Can you work these out from the model? Positions are in its coordinate system, mm. A direction names the side the tool comes from. Round coordinates to 2 decimals unless told otherwise and drop trailing zeros. Write each loop counter-clockwise with the first axis right and the second up, starting at its lowest first coordinate (ties: lowest second). Pieces come first, ordered by that corner, then holes. Notation, with made-up numbers: M 83.5,-25.75 L 109.5,-25.75 A21 cw 109.5,-2.75 Z; hole C 40,34.25 d5. An arc over 180 degrees is marked long. Answer in a Markdown table with one row per item. Add a question column.
(1) Suppose I cut it at B-B, the plane z = 5.3. Write out the boundary of the cut face in (x, y), then the cut area to 3 significant figures.
(2) If I drill on probe 1 along Y at (x, z) = (0, 3.75); probe 2 along Y at (x, z) = (0, 5.75); probe 3 along Z at (x, y) = (-0.2, -17), over which ranges is the centre line in solid material (lowest first)?
(3) If we mould it in two halves opening along X, with no side actions, what happens to faces 1 (the face through (-0.014, -16.405, 4.844)), 2 (the face through (1, 16, 5)), 3 (the face through (5.65, -1.03, 3.79))? For each: released by +X, released by -X, zero draft, split by the parting line, or undercut.
(4) I'm going to push flat-ended pins straight in: pin 1 (2.5 mm diameter, centred on x = 0, y = -6, fed in from +Z); pin 2 (3 mm diameter, centred on x = 0, y = 7, fed in from +Z); pin 3 (2 mm diameter, centred on y = -7.5, z = 5.5, fed in from +X); pin 4 (1.7 mm diameter, centred on y = 17, z = 5.3, fed in from +X). Where does each tip first touch, or does it pass through?
(5) For faces 4 (the face through (15, 0, 7)), 5 (the face through (-1, -16, 5)), 6 (the face through (0.585, -4.364, 6.279)), which set-ups out of +Z, -Z, +X, -X, +Y, -Y let a thin tool reach every point of the face, with its end or its side?
(6) Suppose I cut it at A-A, the plane x = 0. Write out the boundary of the cut face in (y, z).
from build123d import *

# Parameters (mm, degrees)
SKETCH050_R             = 15
SKETCH050_R_2           = 2.75
SKETCH050_R_3           = 1.7
PAD021_DEPTH            = 5
SKETCH051_R             = 2.7
POCKET026_DEPTH         = 88.441037
POLARPATTERN004_COUNT   = 4
PAD022_DEPTH            = 5
SKETCH054_R             = 0.75
POCKET027_DEPTH         = 5
POLARPATTERN005_COUNT   = 2
BODY011_PLACEMENT_ANGLE = 270


with BuildPart() as part:
    # Sketch050 → Pad021 (new body)
    with BuildSketch(Plane.XZ):
        Circle(SKETCH050_R)
        Circle(SKETCH050_R_2, mode=Mode.SUBTRACT)
        with Locations((0, 7)):
            Circle(SKETCH050_R_3, mode=Mode.SUBTRACT)
        with Locations((-7, 0)):
            Circle(SKETCH050_R_3, mode=Mode.SUBTRACT)
        with Locations((0, -7)):
            Circle(SKETCH050_R_3, mode=Mode.SUBTRACT)
        with Locations((7, 0)):
            Circle(SKETCH050_R_3, mode=Mode.SUBTRACT)
    extrude(amount=PAD021_DEPTH)

    # Sketch051 → Pocket026 (cut, through all)
    with BuildSketch(Plane.XZ.offset(2)):
        with Locations((0, 7)):
            Circle(SKETCH051_R)
    pocket026 = extrude(amount=POCKET026_DEPTH, mode=Mode.SUBTRACT)

    # PolarPattern004: Pocket026 ×4 about axis
    polarpattern004_axis = Axis((0, -2, 0), (0, -1, 0))
    for i in range(1, POLARPATTERN004_COUNT):
        add(pocket026.rotate(polarpattern004_axis, i * 360 / POLARPATTERN004_COUNT), mode=Mode.SUBTRACT)

    # Sketch052 → Groove003 (revolve, cut)
    with BuildSketch(Plane.YZ):
        with BuildLine():
            ThreePointArc((-4, 15), (-2.5, 14.197224), (-1, 15))
            Line((-4, 15), (-1, 15))
        make_face()
    revolve(axis=Axis((0, 0, 0), (0, 1, 0)), mode=Mode.SUBTRACT)

    # Sketch053 (on Face10 of Groove003) → Pad022 (join)
    with BuildSketch(Plane.XZ.offset(5)):
        with BuildLine():
            ThreePointArc((1, 18), (0, 19), (-1, 18))
            Line((-1, 18), (-1, 10))
            Line((-1, 10), (1, 10))
            Line((1, 10), (1, 18))
        make_face()
    pad022 = extrude(amount=-PAD022_DEPTH)

    # Sketch054 (on Face6 of Pad022) → Pocket027 (cut)
    with BuildSketch(Plane(origin=(1, 0, 0), x_dir=(0, 0, 1), z_dir=(1, 0, 0))):
        with Locations((17, 2.5)):
            Circle(SKETCH054_R)
    pocket027 = extrude(amount=-POCKET027_DEPTH, mode=Mode.SUBTRACT)

    # PolarPattern005: Pad022, Pocket027 ×2 about axis
    polarpattern005_axis = Axis((0, -5, 0), (0, -1, 0))
    for i in range(1, POLARPATTERN005_COUNT):
        add(pad022.rotate(polarpattern005_axis, i * 360 / POLARPATTERN005_COUNT))
        add(pocket027.rotate(polarpattern005_axis, i * 360 / POLARPATTERN005_COUNT), mode=Mode.SUBTRACT)


with BuildPart() as part_1:
    # Body011 placement: moved
    add(part.part.moved(Location((0, 0, 2.8))).rotate(Axis((0, 0, 2.8), (1, 0, 0)), BODY011_PLACEMENT_ANGLE))


solid = part_1.part
Calculated:
| question | item | result |
|---|---|---|
| 1 | outline | M -1,-18 A1 ccw 1,-18 L 1,-17.75 L -1,-17.75 Z; M -1,-16.25 L 1,-16.25 L 1,-14.16 A14.2 ccw 1,14.16 L 1,16.25 L -1,16.25 L -1,14.16 A14.2 ccw -1,-14.16 Z; M -1,17.75 L 1,17.75 L 1,18 A1 ccw -1,18 Z; hole C -7,0 d5.4; hole C 0,0 d5.5; hole C 0,-7 d5.4; hole C 0,7 d5.4; hole C 7,0 d5.4 |
| 1 | area | 530 mm² |
| 2 | probe 1 | -19 to -8.7, -5.3 to -2.75, 2.75 to 5.3, 8.7 to 19 |
| 2 | probe 2 | -19 to -17.6, -16.4 to -9.7, -4.3 to -2.75, 2.75 to 4.3, 9.7 to 16.4, 17.6 to 19 |
| 2 | probe 3 | 2.8 to 4.55, 6.05 to 7.8 |
| 3 | face 1 | zero draft |
| 3 | face 2 | released by +X |
| 3 | face 3 | undercut |
| 4 | pin 1 | z = 4.8 |
| 4 | pin 2 | through |
| 4 | pin 3 | x = 12.75 |
| 4 | pin 4 | x = 1 |
| 5 | face 4 | +Z, -Z, +X |
| 5 | face 5 | -X, -Y |
| 5 | face 6 | +Z |
| 6 | outline | M -19,2.8 L -8.7,2.8 L -8.7,4.8 L -9.7,4.8 L -9.7,7.8 L -19,7.8 Z; M -5.3,2.8 L -2.75,2.8 L -2.75,7.8 L -4.3,7.8 L -4.3,4.8 L -5.3,4.8 Z; M 2.75,2.8 L 5.3,2.8 L 5.3,4.8 L 4.3,4.8 L 4.3,7.8 L 2.75,7.8 Z; M 8.7,2.8 L 19,2.8 L 19,7.8 L 9.7,7.8 L 9.7,4.8 L 8.7,4.8 Z; hole C -17,5.3 d1.5; hole C 17,5.3 d1.5 |
